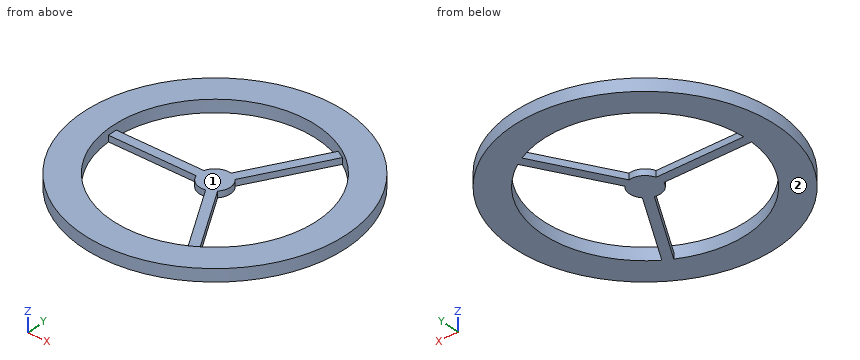
from build123d import *

# Parameters (mm, degrees)
SKETCH1_R           = 42.5
BOSS_EXTRUDE1_DEPTH = 4
SKETCH3_R           = 33
SKETCH3_R_2         = 5
CUT_EXTRUDE2_DEPTH  = 61.237031799
SKETCH4_W           = 35
SKETCH4_H           = 3
BOSS_EXTRUDE3_DEPTH = 4
SKETCH5_R           = 33
CUT_EXTRUDE4_DEPTH  = 2


# Read off the part's stored shape, not the designer's step: Cavity1
with BuildPart() as part:
    # Sketch1 → Boss-Extrude1 (new body)
    with BuildSketch(Plane.XY):
        Circle(SKETCH1_R)
    extrude(amount=BOSS_EXTRUDE1_DEPTH)

    # Cavity1 outline → Cavity1 (revolve, cut)
    with BuildSketch(Plane.XZ):
        Polygon((0.75, 0), (0.75, 3.9), (0.65, 4), (0, 4), (0, 0), align=None)
    revolve(axis=Axis((0, 0, 0), (0, 0, 1)), mode=Mode.SUBTRACT)

    # Sketch3 → Cut-Extrude2 (cut, through all)
    with BuildSketch(Plane.XY.offset(4)):
        Circle(SKETCH3_R)
        Circle(SKETCH3_R_2, mode=Mode.SUBTRACT)
    extrude(amount=-CUT_EXTRUDE2_DEPTH, mode=Mode.SUBTRACT)


with BuildPart() as cut_extrude2_piece_1:
    # of the separate pieces the step leaves, piece 1, a body of its own (cut_extrude2_pieces)
    add(part.part.solids().sort_by_distance((42.5, 0, 0))[0])



with BuildPart() as cut_extrude2_piece_2:
    # of the separate pieces the step leaves, piece 2, a body of its own (cut_extrude2_pieces)
    add(part.part.solids().sort_by_distance((5, 0, 0))[0])


with BuildPart() as cut_extrude2_piece_1_1:
    add(cut_extrude2_piece_1.part)

    add(cut_extrude2_piece_2.part)  # Boss-Extrude3 merges Cut-Extrude2 piece 2
    # Sketch4 → Boss-Extrude3 (add)
    with BuildSketch(Plane.XY.offset(4)):
        with Locations((-17.5, 0)):
            Rectangle(SKETCH4_W, SKETCH4_H)
        Polygon((-1.299038106, 0.75), (16.200961894, 31.060889132), (18.799038106, 29.560889132), (1.299038106, -0.75), align=None)
        Polygon((1.299038106, 0.75), (18.799038106, -29.560889132), (16.200961894, -31.060889132), (-1.299038106, -0.75), align=None)
    extrude(amount=-BOSS_EXTRUDE3_DEPTH)

    # Sketch5 → Cut-Extrude4 (cut)
    with BuildSketch(Plane.XY.offset(4)):
        Circle(SKETCH5_R)
    extrude(amount=-CUT_EXTRUDE4_DEPTH, mode=Mode.SUBTRACT)


solid = cut_extrude2_piece_1_1.part
For this review, take the finished solid that the model builds, in its own axes (mm). Face numbers are marked on the shaded views. Round coordinates to 2 decimals unless told otherwise and drop trailing zeros. Loops run counter-clockwise (first coordinate to the right, second up) from the corner with the lowest first, then second, coordinate; pieces in that order, holes last. Notation, with made-up numbers: (51, 79) - (55, 79) arc R18 ccw to (55, 107) - close; hole circle Ø2 at (29, 42). An arc over 180 degrees is marked (long way). One line per item, written item: value. Start each with the question number.
Item 1: Clearance check with flat-ended pins moving along their axes: pin 1 Ø1 at (y, z) = (-33.5, 1) entering from +X; pin 2 Ø15 at (x, y) = (-2.5, -14.5) entering from +Z; pin 3 Ø2 at (x, z) = (5.5, 3) entering from +Y; pin 4 Ø1.6 at (x, z) = (-17.5, 1) entering from +Y. State where each tip first meets the part, or that it passes through.
Item 2: The part is to be moulded in two halves that separate along Y. For the marked faces 1 and 2, say which applies: +Y half, -Y half, draft (parallel to the pull), parting line (faces both ways), or undercut.
Item 3: Take a section at A-A (y = 0). Give the boundary of the cut face in (x, z), plus the area to 3 significant figures.
Item 4: Take a section at B-B (x = 0). Give the boundary of the cut face in (y, z).
Item 5: Take a section at C-C (z = 2.95). Give the boundary of the cut face in (x, y), plus the area to 3 significant figures.
Item 6: For L1, parallel to Y at x = 0, z = 1.1; L2, parallel to Y at x = 0, z = 2.8; L3, parallel to X at y = -20, z = 1.75, list the stretches that pass through material, from the lowest coordinate up.
Item 7: Take a section at D-D (x = 28). Give the boundary of the cut face in (y, z), plus the area to 3 significant figures.
Answer below:
1. pin 1: stops at x = 26.78
1. pin 2: passes through
1. pin 3: stops at y = 42.26
1. pin 4: stops at y = 39.08
2. face 1: undercut
2. face 2: draft
3. outline: (-42.5, 0) - (5, 0) - (5, 2) - (-33, 2) - (-33, 4) - (-42.5, 4) - close; (33, 0) - (42.5, 0) - (42.5, 4) - (33, 4) - close
3. area: 152 mm2
4. outline: (-42.5, 0) - (-33, 0) - (-33, 4) - (-42.5, 4) - close; (-5, 0) - (5, 0) - (5, 2) - (-5, 2) - close; (33, 0) - (42.5, 0) - (42.5, 4) - (33, 4) - close
5. outline: circle Ø85 at (0, 0); hole circle Ø66 at (0, 0)
5. area: 2,250 mm2
6. L1: y = -42.5 to -33, -5 to 5, 33 to 42.5
6. L2: y = -42.5 to -33, 33 to 42.5
6. L3: x = -37.5 to -26.25, 9.81 to 13.28, 26.25 to 37.5
7. outline: (-31.97, 0) - (-17.46, 0) - (-17.46, 4) - (-31.97, 4) - close; (17.46, 0) - (31.97, 0) - (31.97, 4) - (17.46, 4) - close
7. area: 116 mm2
